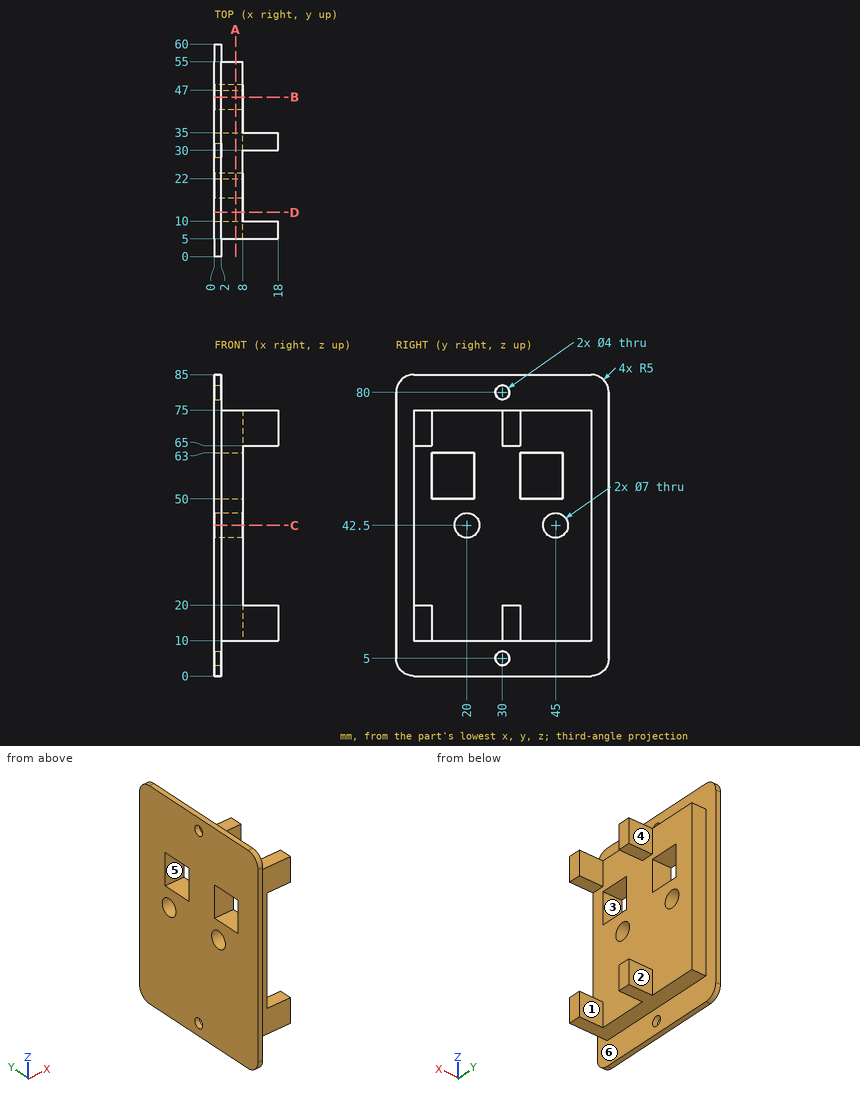
Answer from the drawing. Dimensions are ordinates in mm from the lowest x, y and z of the part. A direction names the side the tool comes from. Give positions to 0.01 mm unless a question says otherwise; leave off trailing zeros. Write each loop counter-clockwise with the first axis right and the second up, starting at its lowest first coordinate (ties: lowest second). Pieces come first, ordered by that corner, then holes.
1) For a pull along Y with two mould halves and no side action, classify the marked faces 4, 5 and 6 as pulls with the +Y half, pulls with the -Y half, needs draft (parallel to the pull), parting line crosses it, or undercut.
2) Section D-D (y = 12.5) is taken. Write down the section's boundary in (x, z), and give its area (3 significant figures).
3) A tool of negligible diameter and unlimited length cuts with its end or side. For the marked faces 1, 2 and 3, from which of +Z, -Z, +X, -X, +Y, -Y can it reach the whole face along a straight path? Write none if from no direction.
4) Section A-A (x = 6) is taken. Write down the section's boundary in (y, z), and give its area (3 significant figures).
5) Find the intervals of material crossed by L1, parallel to Y at x = 6, z = 51; L2, parallel to Y at x = 5, z = 42.5; L3, parallel to Z at x = 1.1, y = 30, in increasing order.
6) Given P1, Ø4, axis at x = 12, y = 7.5, coming from the +Z side; P2, Ø5.5, axis at x = 14, y = 32.5, coming from the -Z side; P3, Ø10, axis at y = 7.5, z = 50.5, coming from the +X side, each flat-ended and moving along its own axis, determine where each tip first touches the part or whether it passes through.
7) Section B-B (y = 45) is taken. Write down the section's boundary in (x, z).
8) Section C-C (z = 42.5) is taken. Write down the section's boundary in (x, y), and give its area (3 significant figures).
Response:
1. face 4: pulls with the +Y half
1. face 5: undercut
1. face 6: needs draft
2. outline: (0, 0) - (2, 0) - (2, 10) - (8, 10) - (8, 50) - (0, 50) - close; (0, 63) - (8, 63) - (8, 75) - (2, 75) - (2, 85) - (0, 85) - close
2. area: 456 mm2
3. face 1: +Z, -Z, +X
3. face 2: +Z, -Z, +X, +Y
3. face 3: +X, -X
4. outline: (5, 10) - (55, 10) - (55, 75) - (5, 75) - close; hole (10, 50) - (22, 50) - (22, 63) - (10, 63) - close; hole circle Ø7 at (20, 42.5); hole (35, 50) - (47, 50) - (47, 63) - (35, 63) - close; hole circle Ø7 at (45, 42.5)
4. area: 2,860 mm2
5. L1: y = 5 to 10, 22 to 35, 47 to 55
5. L2: y = 5 to 16.5, 23.5 to 41.5, 48.5 to 55
5. L3: z = 0 to 3, 7 to 78, 82 to 85
6. P1: stops at z = 75
6. P2: stops at z = 10
6. P3: stops at x = 8
7. outline: (0, 0) - (2, 0) - (2, 10) - (8, 10) - (8, 39) - (0, 39) - close; (0, 46) - (8, 46) - (8, 50) - (0, 50) - close; (0, 63) - (8, 63) - (8, 75) - (2, 75) - (2, 85) - (0, 85) - close
8. outline: (0, 0) - (2, 0) - (2, 5) - (8, 5) - (8, 16.5) - (0, 16.5) - close; (0, 23.5) - (8, 23.5) - (8, 41.5) - (0, 41.5) - close; (0, 48.5) - (8, 48.5) - (8, 55) - (2, 55) - (2, 60) - (0, 60) - close
8. area: 308 mm2
